Autodesk Inventor part; units mm, degrees
ref_plane "YZ Plane" through (0, 0, 0) normal (1, 0, 0) x (0, 1, 0)
ref_plane "XZ Plane" through (0, 0, 0) normal (0, 1, 0) x (-1, 0, 0)
ref_plane "XY Plane" through (0, 0, 0) normal (0, 0, 1) x (1, 0, 0)
sketch "スケッチ1" plane through (0, 0, 0) normal (0, 1, 0) x (-1, 0, 0)
  line L0 (0, 99) -> (20, 99)
  line L1 (20, 99) -> (20, -99)
  line L2 (20, -99) -> (0, -99)
  line L3 (0, -99) -> (0, 99)
  point P0 (0, 0)
  point P1 (0, 0)
  dimension "d0" = 198
  dimension "d1" = 20
extrude "押し出し1" add sketch "スケッチ1" along normal blind 5.5
sketch "スケッチ2" plane through (0, 5.5, 0) normal (0, 1, 0) x (1, 0, 0)
  line L0 (-15, -67.8) -> (-5, -67.8)
  line L1 (-5, -67.8) -> (-5, -64.8)
  line L2 (-5, -64.8) -> (-15, -64.8)
  line L3 (-15, -64.8) -> (-15, -67.8)
  line L4 (-8.5, -71.3) -> (-11.5, -71.3)
  line L5 (-11.5, -71.3) -> (-11.5, -61.3)
  line L6 (-11.5, -61.3) -> (-8.5, -61.3)
  line L7 (-8.5, -61.3) -> (-8.5, -71.3)
  line L8 (-20, -99) -> (0, -99)
  circle A0 centre (-10, -94.3) radius 1.6
  point P0 (0, 0)
  point P1 (-8.5, -66.3)
  point P2 (-15, -66.3)
  point P3 (-10, -71.3)
  point P4 (-10, -67.8)
  point P5 (-10, -99)
  point P6 (-8.5, -64.8)
  point P7 (-11.5, -64.8)
  point P8 (-11.5, -67.8)
  point P9 (-8.5, -67.8)
  point P10 (-10, -99)
  dimension "d4" = 10
  dimension "d5" = 27.7
  dimension "d6" = 3
  dimension "d9" = 3.2
  dimension "d10" = 4.7
extrude "押し出し2" cut sketch "スケッチ2" against normal through all
mirror "ミラー1" about plane through (0, 0, 0) normal (0, 0, 1) of "押し出し2"
properties part number "front_connector_base" material "木材 (カエデ材)"
Verification items for the finished model (mm, model axes). Coordinates: 2 decimals unless noted, no trailing zeros. Write each loop counter-clockwise with the first axis right and the second up, starting at its lowest first coordinate (ties: lowest second). Pieces come first, ordered by that corner, then holes. Notation, with made-up numbers: M -32.5,14 L 1.5,14 A25 ccw 1.5,31 Z; hole C 86.25,-14.75 d10. An arc over 180 degrees is marked long. One line per question, with ' | ' between items.
1) Depth check by flat-ended pin: pin 1 Ø3 at (x, z) = (-10, -94.3) entering from +Y. Enter the tip coordinate at first touch or a pass-through.
Solutions:
pin 1: through
2) Material ranges on L1, parallel to Z at x = -10, y = 3.75; L2, parallel to Z at x = -8, y = 1.2; L3, parallel to X at y = 3.8, z = -94.3, recorded low to high.
Solutions:
L1: -99 to -95.9, -92.7 to -71.3, -61.3 to 61.3, 71.3 to 92.7, 95.9 to 99 | L2: -99 to -67.8, -64.8 to 64.8, 67.8 to 99 | L3: -20 to -11.6, -8.4 to 0
3) Sectioned sample at A-A on z = -94.3. Record the cut outline in (x, y), then the cut area to 3 significant figures.
Solutions:
outline: M -20,0 L -11.6,0 L -11.6,5.5 L -20,5.5 Z; M -8.4,0 L 0,0 L 0,5.5 L -8.4,5.5 Z | area: 92.4 mm^2
4) Release check for a two-part mould opening along Z. For faces 1 (the face through (-7, 3, -67.8)), 2 (the face through (-13, 3, 67.8)), 3 (the face through (-20, 3, 1)) record: +Z half, -Z half, draft (parallel to the pull), parting line (faces both ways), or undercut.
Solutions:
face 1: undercut | face 2: undercut | face 3: draft
5) Sectioned sample at B-B on y = 1.35. State how many separate pieces and enclosed holes the cut face has, then the cut area to 3 significant figures.
Solutions:
separate pieces: 1 | enclosed holes: 4 | area: 3,840 mm^2
